Input: part model. Units: mm. Frame: model coordinates. Coordinates: 2 decimals unless noted, no trailing zeros. Order: outer loops, then holes, each group sorted by start corner. A loop starts at its lowest first (then second) coordinate and runs counter-clockwise, first axis right, second up.
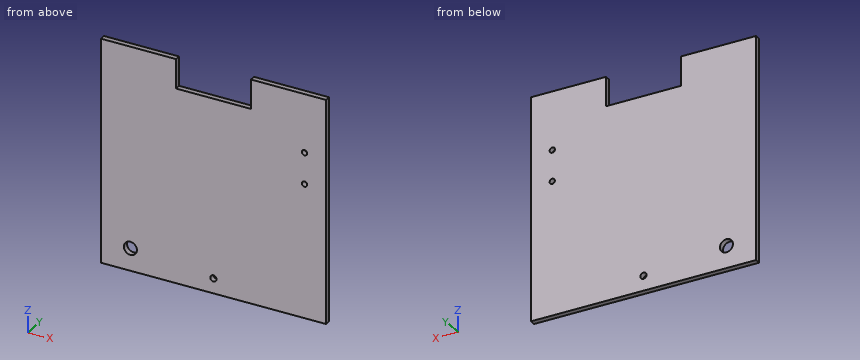
from build123d import *

# Parameters (mm, degrees)
SKETCH1_W           = 193.68
SKETCH1_H           = 190.5
BOSS_EXTRUDE1_DEPTH = 4.78
SKETCH2_R           = 2.6797
CUT_EXTRUDE1_DEPTH  = 5.78
CUT_EXTRUDE2_DEPTH  = 5.78
SKETCH5_R           = 2.286
SKETCH5_R_2         = 5.6134
CUT_EXTRUDE3_DEPTH  = 5.78


with BuildPart() as part:
    # Sketch1 → Boss-Extrude1 (new body)
    with BuildSketch(Plane(origin=(0, 0, 0), x_dir=(1, 0, 0), z_dir=(0, 1, 0))):
        Rectangle(SKETCH1_W, SKETCH1_H)
    extrude(amount=BOSS_EXTRUDE1_DEPTH)

    # Sketch2 → Cut-Extrude1 (cut, through all)
    with BuildSketch(Plane(origin=(0, 4.78, 0), x_dir=(1, 0, 0), z_dir=(0, 1, 0))):
        with Locations((0, 82.55)):
            Circle(SKETCH2_R)
    extrude(amount=-CUT_EXTRUDE1_DEPTH, mode=Mode.SUBTRACT)

    # Sketch3 → Cut-Extrude2 (cut, through all)
    with BuildSketch(Plane(origin=(0, 4.78, 0), x_dir=(1, 0, 0), z_dir=(0, 1, 0))):
        Polygon((0, -95.25), (-32.28, -95.25), (-32.28, -70.249999962), (32.28, -70.249999962), (32.28, -95.25), align=None)
    extrude(amount=-CUT_EXTRUDE2_DEPTH, mode=Mode.SUBTRACT)

    # Sketch5 → Cut-Extrude3 (cut, through all)
    with BuildSketch(Plane(origin=(0, 4.78, 0), x_dir=(1, 0, 0), z_dir=(0, 1, 0))):
        with Locations((78.425, -18.77099)):
            Circle(SKETCH5_R)
        with Locations((78.425, -45.44099)):
            Circle(SKETCH5_R)
        with Locations((-71.44, 76.2)):
            Circle(SKETCH5_R_2)
    extrude(amount=-CUT_EXTRUDE3_DEPTH, mode=Mode.SUBTRACT)


solid = part.part
Item 1: Cut plane B-B on z = -76.2. Return loops of the section in (x, y).
Response values:
outline: (-96.84, 0) - (-77.05, 0) - (-77.05, 4.78) - (-96.84, 4.78) - close; (-65.83, 0) - (96.84, 0) - (96.84, 4.78) - (-65.83, 4.78) - close
Item 2: Ray query, probe 1 along X at (y, z) = (3.6, 70.5); probe 2 along Z at (x, y) = (0, 3.2); probe 3 along Z at (x, y) = (-71.44, 1.9). Return the intervals inside material, ascending.
Response values:
probe 1: x = -96.84 to -32.28, 32.28 to 96.84
probe 2: z = -95.25 to -85.23, -79.87 to 70.25
probe 3: z = -95.25 to -81.81, -70.59 to 95.25
Item 3: Pin query (flat end, axial travel): pin 1 Ø7.5 at (x, z) = (78.42, 18.77) entering from -Y; pin 2 Ø1.5 at (x, y) = (30, 2) entering from +Z. Return the tip coordinate at first contact, or that it passes through.
Response values:
pin 1: stops at y = 0
pin 2: stops at z = 70.25
Item 4: Cut plane D-D on x = -9. Return loops of the section in (y, z).
Response values:
outline: (0, -95.25) - (4.78, -95.25) - (4.78, 70.25) - (0, 70.25) - close
Item 5: Cut plane A-A on x = -71.44. Return loops of the section in (y, z), then the cut area to 3 significant figures.
Response values:
outline: (0, -95.25) - (4.78, -95.25) - (4.78, -81.81) - (0, -81.81) - close; (0, -70.59) - (4.78, -70.59) - (4.78, 95.25) - (0, 95.25) - close
area: 857 mm2
Item 6: Cut plane C-C on y = 2.1. Return loops of the section in (x, z) (3 decimals).
Response values:
outline: (-96.84, -95.25) - (96.84, -95.25) - (96.84, 95.25) - (32.28, 95.25) - (32.28, 70.25) - (-32.28, 70.25) - (-32.28, 95.25) - (-96.84, 95.25) - close; hole circle Ø11.227 at (-71.44, -76.2); hole circle Ø5.359 at (0, -82.55); hole circle Ø4.572 at (78.425, 18.771); hole circle Ø4.572 at (78.425, 45.441)
